Check sheet for the drawn part. Datum: minimum x, y, z corner. Units: mm. A direction names the side the tool comes from. Coordinates: 2 decimals unless noted, no trailing zeros. Write each loop counter-clockwise with the first axis right and the second up, starting at its lowest first coordinate (ties: lowest second). Pieces come first, ordered by that corner, then holes. Notation, with made-up numbers: (68.5, -36.75) -> (122.5, -36.75) arc R26 cw to (122.5, 0.25) -> close; hole circle Ø1 at (-3.75, 2.5). An arc over 180 degrees is marked (long way). Write item = value, one per line. Start each with the question number.
(1) Section check A-A (x = 16). Record the cut outline in (y, z).
(2) Section check D-D (y = 2). Record the cut outline in (x, z), plus the area to 3 significant figures.
(3) Section check B-B (y = 22). Record the cut outline in (x, z), plus the area to 3 significant figures.
(4) Material ranges on probe 1 along Y at (x, z) = (16, 2); probe 2 along Z at (x, y) = (21, 29.5); probe 3 along X at (y, z) = (7, 1.5), recorded low to high. Write a range as [from, to].
(5) Set-up check for the marked faces 1, 2 and 3: record each of +Z, -Z, +X, -X, +Y, -Y from which the full face is reachable in a straight line by a thin tool's end or side.
(6) Mould release check, pull along Y, two halves, no side actions. Record for the marked faces 4, 5 and 6: released by +Y, released by -Y, zero draft, split by the parting line, or undercut.
(7) Section check C-C (z = 3). Record the cut outline in (x, y).
(8) Gauge pin test, flat ends, axial feed: pin 1 Ø6 at (x, y) = (7, 21.5) entering from -Z; pin 2 Ø4 at (x, z) = (22.5, 4) entering from +Y; pin 3 Ø4 at (x, z) = (27, 4.5) entering from -Y; pin 4 Ø3 at (x, z) = (18, 6) entering from -Y. Record the tip position at first contact, or that the pin passes through.
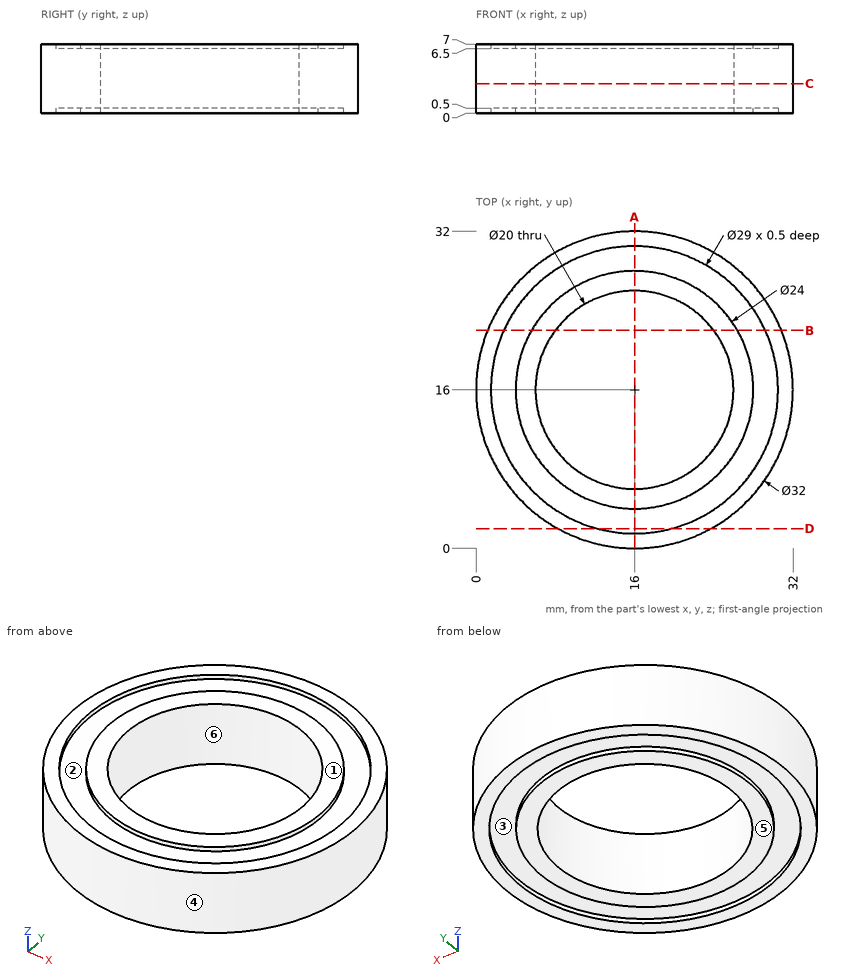
Response:
q1.outline = (0, 0) -> (1.5, 0) -> (1.5, 0.5) -> (4, 0.5) -> (4, 0) -> (6, 0) -> (6, 7) -> (4, 7) -> (4, 6.5) -> (1.5, 6.5) -> (1.5, 7) -> (0, 7) -> close; (26, 0) -> (28, 0) -> (28, 0.5) -> (30.5, 0.5) -> (30.5, 0) -> (32, 0) -> (32, 7) -> (30.5, 7) -> (30.5, 6.5) -> (28, 6.5) -> (28, 7) -> (26, 7) -> close
q2.outline = (8.25, 0) -> (12.23, 0) -> (12.23, 0.5) -> (19.77, 0.5) -> (19.77, 0) -> (23.75, 0) -> (23.75, 7) -> (19.77, 7) -> (19.77, 6.5) -> (12.23, 6.5) -> (12.23, 7) -> (8.25, 7) -> close
q2.area = 101 mm2
q3.outline = (1.17, 0) -> (2.8, 0) -> (2.8, 0.5) -> (5.61, 0.5) -> (5.61, 0) -> (8, 0) -> (8, 7) -> (5.61, 7) -> (5.61, 6.5) -> (2.8, 6.5) -> (2.8, 7) -> (1.17, 7) -> close; (24, 0) -> (26.39, 0) -> (26.39, 0.5) -> (29.2, 0.5) -> (29.2, 0) -> (30.83, 0) -> (30.83, 7) -> (29.2, 7) -> (29.2, 6.5) -> (26.39, 6.5) -> (26.39, 7) -> (24, 7) -> close
q3.area = 90.0 mm2
q4.probe_1 = [0, 6], [26, 32]
q4.probe_2 = [0.5, 6.5]
q4.probe_3 = [2.77, 11.64], [20.36, 29.23]
q5.face_1 = +Z, +X, -X, +Y, -Y
q5.face_2 = +Z
q5.face_3 = -Z
q6.face_4 = split by the parting line
q6.face_5 = zero draft
q6.face_6 = undercut
q7.outline = circle Ø32 at (16, 16); hole circle Ø20 at (16, 16)
q8.pin_1 = 0
q8.pin_2 = 31.35
q8.pin_3 = 2.77
q8.pin_4 = 0.01
